from build123d import *

# Parameters (mm, degrees)
SKETCH_1_R      = 7.94
SKETCH_1_R_2    = 1.697891057
SKETCH_1_R_3    = 1.431269813
EXTRUDE_1_DEPTH = 5


with BuildPart() as part:
    # 草图1 → 凸台-拉伸1 (new body)
    with BuildSketch(Plane.XY):
        with BuildLine():
            Line((-22.842936614, 35.573770492), (-22.842936614, -16.926229508))
            ThreePointArc((-22.842936614, -16.926229508), (-5.342936614, -34.426229508), (12.157063386, -16.926229508))
            Line((12.157063386, -16.926229508), (12.157063386, 35.573770492))
            ThreePointArc((12.157063386, 35.573770492), (8.922010957, 38.80882292), (5.686958528, 35.573770492))
            ThreePointArc((5.686958528, 35.573770492), (-5.342936614, 24.543875349), (-16.372831757, 35.573770492))
            ThreePointArc((-16.372831757, 35.573770492), (-19.607884186, 38.80882292), (-22.842936614, 35.573770492))
        make_face()
        with Locations((-5.342936614, -16.926229508)):
            Circle(SKETCH_1_R, mode=Mode.SUBTRACT)
        with Locations((-19.607884186, 35.573770492)):
            Circle(SKETCH_1_R_2, mode=Mode.SUBTRACT)
        with Locations((8.922010957, 35.573770492)):
            Circle(SKETCH_1_R_2, mode=Mode.SUBTRACT)
        with Locations((-9.369105652, -6.944867305)):
            Circle(SKETCH_1_R_3, mode=Mode.SUBTRACT)
        with Locations((-15.286101655, -12.698452236)):
            Circle(SKETCH_1_R_3, mode=Mode.SUBTRACT)
        with Locations((-0.625126274, -26.940078994)):
            Circle(SKETCH_1_R_3, mode=Mode.SUBTRACT)
        with Locations((-15.286101655, -21.484473196)):
            Circle(SKETCH_1_R_3, mode=Mode.SUBTRACT)
        with Locations((-9.369105652, -26.940078994)):
            Circle(SKETCH_1_R_3, mode=Mode.SUBTRACT)
        with Locations((-0.625126274, -6.944867305)):
            Circle(SKETCH_1_R_3, mode=Mode.SUBTRACT)
        with Locations((4.733813833, -12.698452236)):
            Circle(SKETCH_1_R_3, mode=Mode.SUBTRACT)
        with Locations((4.733813833, -21.484473196)):
            Circle(SKETCH_1_R_3, mode=Mode.SUBTRACT)
    extrude(amount=EXTRUDE_1_DEPTH)


solid = part.part
Check sheet for the modelled part. Datum: model origin and axes. Units: mm. Give positions to 0.01 mm unless a question says otherwise; leave off trailing zeros. Loops run counter-clockwise (first coordinate to the right, second up) from the corner with the lowest first, then second, coordinate; pieces in that order, holes last. Notation, with made-up numbers: M 67.25,36 L 101.25,36 A15 ccw 101.25,61 Z; hole C 73.25,62 d8. An arc over 180 degrees is marked long. Use a Markdown table: item, result. Add a question column.
Q1. Sectioned sample at D-D, the plane z = 3.05. Give the number of separate pieces and of enclosed holes in the cut face, then the cut area to 3 significant figures.
Q2. Sectioned sample at C-C, the plane x = -1. Record the cut outline in (y, z).
Q3. Sectioned sample at A-A, the plane x = 4. Record the cut outline in (y, z), then the cut area to 3 significant figures.
Q4. Go/stop test with flat-tipped pins: pin 1 (4.5 mm diameter, centred on x = -9.37, y = -6.94, fed in from +Z); pin 2 (1 mm diameter, centred on x = 3, z = 0.5, fed in from +Y); pin 3 (2 mm diameter, centred on x = -10.5, z = 2, fed in from +Y). Record where each tip stops, or that it passes through.
Q5. Sectioned sample at B-B, the plane y = 31. Record the cut outline in (x, z), then the cut area to 3 significant figures.
Q6. Scan lines: line 1 along X through (y, z) = (-13, 1); line 2 along Y through (x, z) = (-9, 1.4); line 3 along X through (y, z) = (-22, 0.3). Record each from-to range of solid material in increasing order. Write a range as [from, to].
Q7. Mould release check, pull along X, two halves, no side actions. Record for faces 1 (the flat face through (-6, 3, 5)), 2 (the cylindrical face through (-13.964, -22.033, 2.465)), 3 (the cylindrical face through (-5.73, -34.42, 2.46)): pulls with the +X half, pulls with the -X half, needs draft (parallel to the pull), parting line crosses it, or undercut.
Verdict:
| question | item | result |
|---|---|---|
| 1 | separate pieces | 1 |
| 1 | enclosed holes | 11 |
| 1 | area | 1,890 mm^2 |
| 2 | outline | M -33.88,0 L -28.32,0 L -28.32,5 L -33.88,5 Z; M -25.56,0 L -23.57,0 L -23.57,5 L -25.56,5 Z; M -10.28,0 L -8.33,0 L -8.33,5 L -10.28,5 Z; M -5.56,0 L 25.43,0 L 25.43,5 L -5.56,5 Z |
| 3 | outline | M -31.72,0 L -22.71,0 L -22.71,5 L -31.72,5 Z; M -20.26,0 L -13.93,0 L -13.93,5 L -20.26,5 Z; M -11.47,0 L 29.71,0 L 29.71,5 L -11.47,5 Z |
| 3 | area | 283 mm^2 |
| 4 | pin 1 | z = 5 |
| 4 | pin 2 | y = 28.98 |
| 4 | pin 3 | y = 26.42 |
| 5 | outline | M -22.84,0 L -15.38,0 L -15.38,5 L -22.84,5 Z; M 4.69,0 L 12.16,0 L 12.16,5 L 4.69,5 Z |
| 5 | area | 74.6 mm^2 |
| 6 | line 1 | [-22.84, -16.69], [-13.89, -12.24], [1.56, 3.33], [6.13, 12.16] |
| 6 | line 2 | [-34.04, -28.32], [-25.56, -23.97], [-9.88, -8.33], [-5.56, 25.17] |
| 6 | line 3 | [-22.09, -16.62], [-13.95, -11.45], [0.76, 3.4], [6.07, 11.41] |
| 7 | face 1 | needs draft |
| 7 | face 2 | undercut |
| 7 | face 3 | parting line crosses it |
